from build123d import *

# Parameters (mm, degrees)
SKETCH_1_W          = 6
SKETCH_1_H          = 6
EXTRUDE_2_DEPTH     = 6
SKETCH_6_R          = 1.6
CUT_EXTRUDE_5_DEPTH = 6
SKETCH_7_R          = 1.6
CUT_EXTRUDE_6_DEPTH = 6
SKETCH_8_R          = 1.6
CUT_EXTRUDE_7_DEPTH = 6
SKETCH_9_R          = 5.65
CUT_EXTRUDE_9_DEPTH = 6


with BuildPart() as part:
    # 草图1 → 凸台-拉伸2 (new body)
    with BuildSketch(Plane(origin=(0, 0, 0), x_dir=(1, 0, 0), z_dir=(0, 1, 0))):
        Polygon((-3, 8.803847577), (-6.464101615, 8.803847577), (-10.856406461, 1.196152423), (-9.124355653, -1.803847577), (-6.124355653, -7), (-4.392304845, -10), (4.392304845, -10), (6.124355653, -7), (9.124355653, -1.803847577), (10.856406461, 1.196152423), (6.464101615, 8.803847577), (3, 8.803847577), align=None)
        Polygon((-9.124355653, -1.803847577), (-14.320508076, -4.803847577), (-11.320508076, -10), (-6.124355653, -7), align=None)
        Polygon((11.320508076, -10), (14.320508076, -4.803847577), (9.124355653, -1.803847577), (6.124355653, -7), align=None)
        with Locations((0, 11.803847577)):
            Rectangle(SKETCH_1_W, SKETCH_1_H)
    extrude(amount=EXTRUDE_2_DEPTH)

    # 草图6 → 切除-拉伸5 (cut)
    with BuildSketch(Plane(origin=(-1.5, 0, -2.598076211), x_dir=(-0.8660254037844386, 0, 0.5000000000000001), z_dir=(-0.5000000000000001, 0, -0.8660254037844386))):
        with Locations((11.803847577, 3)):
            Circle(SKETCH_6_R)
    extrude(amount=-CUT_EXTRUDE_5_DEPTH, mode=Mode.SUBTRACT)

    # 草图7 → 切除-拉伸6 (cut)
    with BuildSketch(Plane(origin=(3, 0, 0), x_dir=(0, 0, -1), z_dir=(1, 0, 0))):
        with Locations((11.803847577, 3)):
            Circle(SKETCH_7_R)
    extrude(amount=-CUT_EXTRUDE_6_DEPTH, mode=Mode.SUBTRACT)

    # 草图8 → 切除-拉伸7 (cut)
    with BuildSketch(Plane(origin=(-1.5, 0, 2.598076211), x_dir=(0.8660254037844387, 0, 0.49999999999999983), z_dir=(-0.49999999999999983, 0, 0.8660254037844387))):
        with Locations((11.803847577, 3)):
            Circle(SKETCH_8_R)
    extrude(amount=-CUT_EXTRUDE_7_DEPTH, mode=Mode.SUBTRACT)

    # 草图9 → 切除-拉伸9 (cut)
    with BuildSketch(Plane.XZ):
        with Locations(Location((0, 0, 0), (0, 0, 270))):
            Circle(SKETCH_9_R)
    extrude(amount=-CUT_EXTRUDE_9_DEPTH, mode=Mode.SUBTRACT)


solid = part.part
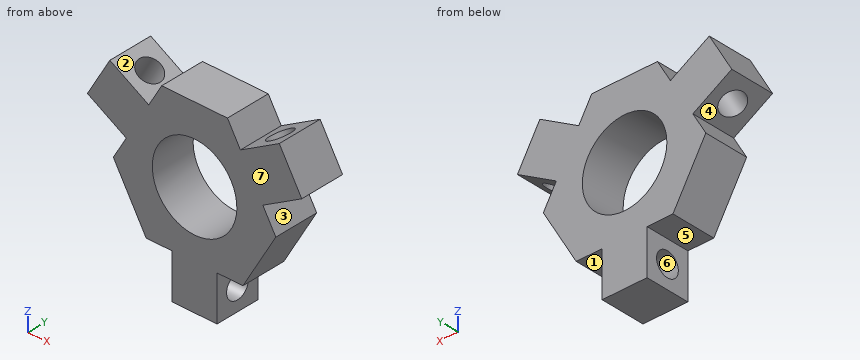
Source: CAD feature listing. Evaluate the final solid. Frame: model axes, mm. Face numbers are marked on the shaded views. A direction names the side the tool comes from. Coordinates: 2 decimals unless noted, no trailing zeros. Order: outer loops, then holes, each group sorted by start corner. A loop starts at its lowest first (then second) coordinate and runs counter-clockwise, first axis right, second up. Notation, with made-up numbers: M 58,-9 L 102,-9 A9 cw 102,7 Z; hole C 51.25,72.25 d4. An arc over 180 degrees is marked long. Write each question's results on one line, items separated by ' | '. Start each with the question number.
1. Pin query (flat end, axial travel): pin 1 (3 mm diameter, centred on y = 3.5, z = -11.5, fed in from -X); pin 2 (1 mm diameter, centred on x = 5.5, y = 4, fed in from -Z); pin 3 (3 mm diameter, centred on y = 4.5, z = -12.5, fed in from +X). Return the tip coordinate at first contact, or that it passes through.
2. Reachability of the marked faces 1, 2, 3 and 4 from +Z, -Z, +X, -X, +Y, -Y: full face, straight path, thin tool, end or side. Return the list, or none.
3. Draft query along Z for the marked faces 5, 6 and 7. Return one class per face: +Z half, -Z half, draft (parallel to the pull), parting line (faces both ways), or undercut.
4. Section B-B, the plane y = 3. State how many separate pieces and enclosed holes the cut face has, then the cut area to 3 significant figures.
5. Section A-A, the plane x = 0. Return the cut outline in (y, z), then the cut area to 3 significant figures.
6. Section D-D, the plane z = -7.25. Return the cut outline in (x, y), then the cut area to 3 significant figures.
7. Material intervals for L1, parallel to X at y = 0.8, z = -9; L2, parallel to Z at x = -2, y = 0.2; L3, parallel to X at y = 3.3, z = 1.75, sorted ascending.
8. Section C-C, the plane z = 0.25. Return the cut outline in (x, y), then the cut area to 3 significant figures.
Solution:
1) pin 1: x = -3 | pin 2: z = -8.8 | pin 3: x = 3
2) face 1: -Z, +X, +Y, -Y | face 2: +Z, +Y, -Y | face 3: +X, +Y, -Y | face 4: -X, +Y, -Y
3) face 5: -Z half | face 6: undercut | face 7: draft
4) separate pieces: 4 | enclosed holes: 1 | area: 253 mm²
5) outline: M 0,-14.8 L 6,-14.8 L 6,-5.65 L 0,-5.65 Z; M 0,5.65 L 6,5.65 L 6,10 L 0,10 Z; hole C 3,-11.8 d3.2 | area: 73.0 mm²
6) outline: M -7.36,0 L 7.36,0 L 7.36,6 L -7.36,6 Z | area: 88.3 mm²
7) L1: -3 to 3 | L2: -14.8 to -5.28, 5.28 to 10 | L3: -9.16 to -5.37, 5.37 to 9.16
8) outline: M -10.02,0 L -5.64,0 L -5.64,6 L -10.02,6 Z; M 5.64,0 L 10.02,0 L 10.02,6 L 5.64,6 Z | area: 52.5 mm²
